from build123d import *

# Parameters (mm, degrees)
SKETCH1_R           = 12
SKETCH1_R_2         = 1.05
BOSS_EXTRUDE1_DEPTH = 5
HOLE2_D             = 7
HOLE2_DEPTH         = 8
HOLE2_CBORE_D       = 9
HOLE2_CBORE_DEPTH   = 2.4
SKETCH8_R           = 2.15
CUT_EXTRUDE1_DEPTH  = 3
FILLET1_R           = 1
FILLET2_R           = 1


with BuildPart() as part:
    # Sketch1 → Boss-Extrude1 (new body)
    with BuildSketch(Plane.XY):
        Circle(SKETCH1_R)
        with Locations((0, 8)):
            Circle(SKETCH1_R_2, mode=Mode.SUBTRACT)
        with Locations((8, 0)):
            Circle(SKETCH1_R_2, mode=Mode.SUBTRACT)
        with Locations((0, -8)):
            Circle(SKETCH1_R_2, mode=Mode.SUBTRACT)
    extrude(amount=BOSS_EXTRUDE1_DEPTH)

    # Hole2
    with Locations(Plane.XY.offset(5)):
        with Locations((-6, 0)):
            CounterBoreHole(HOLE2_D / 2, HOLE2_CBORE_D / 2, HOLE2_CBORE_DEPTH, depth=HOLE2_DEPTH)

    # Sketch8 → Cut-Extrude1 (cut)
    with BuildSketch(Plane(origin=(0, 0, 0), x_dir=(-1, 0, 0), z_dir=(0, 0, -1))):
        with Locations((0, 8)):
            Circle(SKETCH8_R)
        with Locations((0, -8)):
            Circle(SKETCH8_R)
        with Locations((-8, 0)):
            Circle(SKETCH8_R)
    extrude(amount=-CUT_EXTRUDE1_DEPTH, mode=Mode.SUBTRACT)

    # Fillet1
    fillet1_edges = [part.edges().sort_by_distance(p)[0] for p in [
        (-2.5, 0, 0),
        (-2.5, 0, 2.6),
    ]]
    fillet(fillet1_edges, radius=FILLET1_R - 0.0001)  # a hair under: the kernel refuses the full size

    # Fillet2
    fillet2_edges = [part.edges().sort_by_distance(p)[0] for p in [
        (-12, 0, 0),
        (-12, 0, 5),
    ]]
    fillet(fillet2_edges, radius=FILLET2_R)


solid = part.part
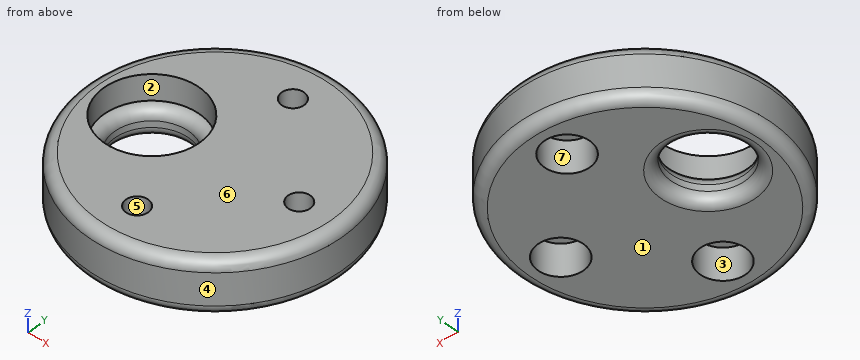
Verification items for the finished model (mm, model axes). Face numbers are marked on the shaded views. A direction names the side the tool comes from. Give positions to 0.01 mm unless a question says otherwise; leave off trailing zeros. Loops run counter-clockwise (first coordinate to the right, second up) from the corner with the lowest first, then second, coordinate; pieces in that order, holes last. Notation, with made-up numbers: (-4, -24.5) - (21, -24.5) arc R8 ccw to (21, -11.5) - close; hole circle Ø5 at (-5.75, -3). An arc over 180 degrees is marked (long way). Write each question's results on one line, items separated by ' | '.
1) Material ranges on L1, parallel to Y at x = 0, z = 4.1; L2, parallel to Y at x = 0, z = 2.25; L3, parallel to Y at x = 8, z = 1.85, recorded low to high. Write a range as from..to.
Solution:
L1: -11.99..-9.05, -6.95..6.95, 9.05..11.99 | L2: -12..-10.15, -5.85..5.85, 10.15..12 | L3: -8.94..-2.15, 2.15..8.94
2) Sectioned sample at A-A on x = 0. Record the boundary of the cut face in (y, z).
Solution:
outline: (-12, 1) arc R1 ccw to (-11, 0) - (-10.15, 0) - (-10.15, 3) - (-9.05, 3) - (-9.05, 5) - (-11, 5) arc R1 ccw to (-12, 4) - close; (-6.95, 3) - (-5.85, 3) - (-5.85, 0) - (5.85, 0) - (5.85, 3) - (6.95, 3) - (6.95, 5) - (-6.95, 5) - close; (9.05, 3) - (10.15, 3) - (10.15, 0) - (11, 0) arc R1 ccw to (12, 1) - (12, 4) arc R1 ccw to (11, 5) - (9.05, 5) - close
3) Sectioned sample at B-B on y = 0. Count the separate pieces of the cut face and the enclosed holes in it, plus the area to 3 significant figures.
Solution:
separate pieces: 3 | enclosed holes: 0 | area: 61.4 mm2
4) Depth check by flat-ended pin: P1, Ø2.5, axis at x = 0, y = -8, coming from the -Z side; P2, Ø1, axis at y = 6.5, z = 1.5, coming from the +X side; P3, Ø1.5, axis at y = -3.5, z = 2.5, coming from the -X side. Enter the tip coordinate at first touch or a pass-through.
Solution:
P1: z = 3 | P2: x = 10.39 | P3: x = -11.68
5) Mould release check, pull along Y, two halves, no side actions. Record for the marked faces 4, 5, 6 and 7: pulls with the +Y half, pulls with the -Y half, needs draft (parallel to the pull), parting line crosses it, or undercut.
Solution:
face 4: parting line crosses it | face 5: undercut | face 6: needs draft | face 7: undercut
6) Tool access check on the marked faces 1, 2 and 3. Record the directions out of +Z, -Z, +X, -X, +Y, -Y that give a thin tool (end or side, any length) a straight path to the whole face; none if there is none.
Solution:
face 1: -Z, +X, -X, +Y, -Y | face 2: +Z | face 3: -Z
